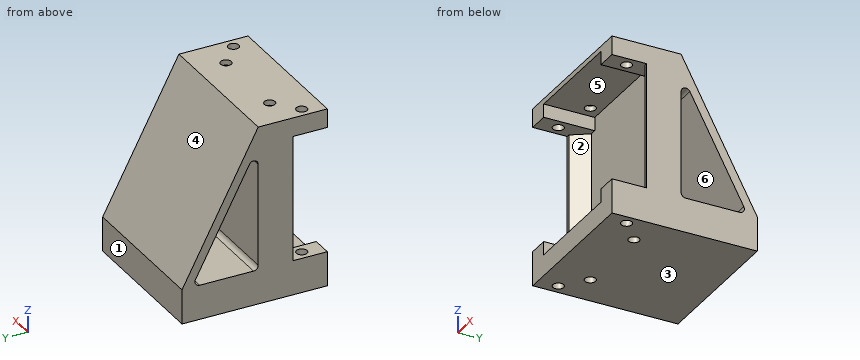
from build123d import *

# Parameters (mm, degrees)
BOSS_EXTRUDE1_DEPTH = 40.132
FILLET1_R           = 1.27
SKETCH2_W           = 28.2956
SKETCH2_H           = 34.036
CUT_EXTRUDE1_DEPTH  = 4.4704
CHAMFER1_SIZE       = 5.08
CHAMFER1_SIZE_2     = 7.53140972
SKETCH3_R           = 1.4605
CUT_EXTRUDE2_DEPTH  = 73.627884767
CUT_EXTRUDE4_REACH  = 76.199
SKETCH4_W           = 28.956
SKETCH4_H           = 41.3004


with BuildPart() as part:
    # Sketch1 → Boss-Extrude1 (new body)
    with BuildSketch(Plane(origin=(0, 0, 0), x_dir=(0, 0, -1), z_dir=(1, 0, 0))):
        Polygon((0, -3.052283086), (0, 36.270517883), (-9.3472, 36.270517883), (-48.4632, 15.642116914), (-48.4632, -3.052283086), (-43.3832, -3.052283086), (-43.3832, 6.294916914), (-9.3472, 6.294916914), (-9.3472, -3.052283086), align=None)
        Polygon((-43.3832, 15.642116914), (-9.3472, 33.59150477), (-9.3472, 15.642116914), align=None, mode=Mode.SUBTRACT)
    extrude(amount=BOSS_EXTRUDE1_DEPTH)

    # Fillet1
    fillet1_edges = [part.edges().sort_by_distance(p)[0] for p in [
        (20.066, 15.642116914, 43.3832),
        (20.066, 15.642116914, 9.3472),
        (20.066, 33.59150477, 9.3472),
    ]]
    fillet(fillet1_edges, radius=FILLET1_R)

    # Sketch2 → Cut-Extrude1 (cut)
    with BuildSketch(Plane.XZ.offset(-6.294916914)):
        with Locations((20.066, 26.3652)):
            Rectangle(SKETCH2_W, SKETCH2_H)
    extrude(amount=-CUT_EXTRUDE1_DEPTH, mode=Mode.SUBTRACT)

    # Chamfer1
    # the kernel refuses this chamfer: 7.53140972, 5.08 mm, written as the material it takes off along each edge
    with BuildSketch(Plane(origin=(5.9182, 6.294916914, 9.3472), x_dir=(-0.9988697089125115, -0.04753214298802862, 0), z_dir=(0, 0, 1))) as chamfer1_piece_1_section:
        Polygon((CHAMFER1_SIZE * 0.998869708913, -CHAMFER1_SIZE * 0.047532142988), (-CHAMFER1_SIZE_2 * 0.0475321429883, -CHAMFER1_SIZE_2 * 0.998869708918), (0, 0), align=None)
    chamfer1_piece_1 = extrude(amount=34.036, mode=Mode.PRIVATE)
    chamfer1_piece_1 = split(chamfer1_piece_1, bisect_by=Plane(origin=(4.025982399, 10.765316914, 26.3652), z_dir=(0, -1, 0)), keep=Keep.TOP, mode=Mode.PRIVATE)
    add(chamfer1_piece_1, mode=Mode.SUBTRACT)
    with BuildSketch(Plane(origin=(34.2138, 6.294916914, 43.3832), x_dir=(0.9988697089125117, -0.0475321429880285, 0), z_dir=(0, 0, -1))) as chamfer1_piece_2_section:
        Polygon((CHAMFER1_SIZE * 0.998869708913, -CHAMFER1_SIZE * 0.047532142988), (-CHAMFER1_SIZE_2 * 0.0475321429883, -CHAMFER1_SIZE_2 * 0.998869708918), (0, 0), align=None)
    chamfer1_piece_2 = extrude(amount=34.036, mode=Mode.PRIVATE)
    chamfer1_piece_2 = split(chamfer1_piece_2, bisect_by=Plane(origin=(36.106017601, 10.765316914, 26.3652), z_dir=(0, -1, 0)), keep=Keep.TOP, mode=Mode.PRIVATE)
    add(chamfer1_piece_2, mode=Mode.SUBTRACT)

    # Sketch3 → Cut-Extrude2 (cut, through all)
    with BuildSketch(Plane(origin=(0, 0, 0), x_dir=(-1, 0, 0), z_dir=(0, 0, -1))):
        with Locations((-37.338, 2.383316914)):
            Circle(SKETCH3_R)
        with Locations((-31.115, 7.717316914)):
            Circle(SKETCH3_R)
        with Locations((-9.017, 7.717316914)):
            Circle(SKETCH3_R)
        with Locations((-2.794, 2.383316914)):
            Circle(SKETCH3_R)
    extrude(amount=-CUT_EXTRUDE2_DEPTH, mode=Mode.SUBTRACT)

    # Cut-Extrude4: up to this face of the body (flat: up to its plane)
    cut_extrude4_end = Plane(part.part.faces().sort_by_distance((20.066, 10.765316914, 26.3652))[0])
    # Sketch4 → Cut-Extrude4 (cut, up to the picked face)
    with BuildSketch(Plane.XZ.offset(3.052283086), mode=Mode.PRIVATE) as cut_extrude4_sk1:
        with Locations((20.066, 26.3652)):
            Rectangle(SKETCH4_W, SKETCH4_H)
    cut_extrude4_tool1 = split(extrude(cut_extrude4_sk1.sketch, amount=-CUT_EXTRUDE4_REACH, mode=Mode.PRIVATE), bisect_by=cut_extrude4_end, keep=Keep.BOTH, mode=Mode.PRIVATE)
    add(cut_extrude4_tool1.solids().sort_by(Axis((20.066, -3.052283, 26.3652), (0, 1, 0)))[0], mode=Mode.SUBTRACT)


solid = part.part
The listing builds one solid part. Answer for the finished solid, in the listing's coordinates (mm). Face numbers are marked on the shaded views. A direction names the side the tool comes from. Give positions to 0.01 mm unless a question says otherwise; leave off trailing zeros. Loops run counter-clockwise (first coordinate to the right, second up) from the corner with the lowest first, then second, coordinate; pieces in that order, holes last. Notation, with made-up numbers: (25.5, 76.25) - (80.5, 76.25) arc R13 cw to (80.5, 99.25) - close; hole circle Ø9 at (19, 80). An arc over 180 degrees is marked (long way). Write each question's results on one line, items separated by ' | '.
1. For a pull along Z with two mould halves and no side action, classify the marked faces 1, 2 and 3 as +Z half, -Z half, draft (parallel to the pull), parting line (faces both ways), or undercut.
Resolved:
face 1: draft | face 2: undercut | face 3: -Z half
2. Consider probe 1 along Z at (x, y) = (27.5, 9) (3 decimals); probe 2 along Y at (x, z) = (15.5, 22); probe 3 along Y at (x, z) = (13, 6). Determine where each line is inside the solid, lowest interval first. Write a range as from..to.
Resolved:
probe 1: z = 0..5.715, 47.015..48.463 | probe 2: y = 10.77..15.64, 26.92..29.6 | probe 3: y = 10.77..36.27
3. Flat-ended cylindrical pins translate along their axes: P1, Ø0.9, axis at x = 39.5, z = 31, coming from the -Y side; P2, Ø8.5, axis at x = 26.5, z = 31, coming from the +Y side; P3, Ø16, axis at x = 22, y = 25, coming from the +Z side. Find the tip coordinate at first contact, or state that the pin passes through.
Resolved:
P1: stops at y = 6.29 | P2: stops at y = 27.09 | P3: stops at z = 45.89
4. Find section C-C, the plane y = 21.5. Write down the section's boundary in (x, z), then the cut area to 3 significant figures.
Resolved:
outline: (0, 0) - (40.13, 0) - (40.13, 9.35) - (0, 9.35) - close; (0, 32.28) - (40.13, 32.28) - (40.13, 37.36) - (0, 37.36) - close | area: 579 mm^2
5. Find section A-A, the plane x = 18.5. Write down the section's boundary in (y, z) (3 decimals), then the cut area to 3 significant figures.
Resolved:
outline: (-3.052, 0) - (36.271, 0) - (36.271, 9.347) - (15.642, 48.463) - (-3.052, 48.463) - (-3.052, 47.015) - (10.765, 47.015) - (10.765, 5.715) - (-3.052, 5.715) - close; hole (15.642, 10.617) arc R1.27 ccw to (16.912, 9.347) - (31.486, 9.347) arc R1.27 ccw to (32.609, 11.21) - (18.035, 38.845) arc R1.27 ccw to (15.642, 38.252) - close | area: 632 mm^2
6. Which of the six approach directions +Z, -Z, +X, -X, +Y, -Y give full straight-line access (tool end or side, diameter ignored) to the marked faces 4, 5 and 6?
Resolved:
face 4: +Z, +X, -X, +Y | face 5: -Y | face 6: +X, -X
7. Find section B-B, the plane z = 37.5. Write down the section's boundary in (x, y).
Resolved:
outline: (0, 6.29) - (0.84, 6.29) - (3.85, 10.77) - (36.28, 10.77) - (39.29, 6.29) - (40.13, 6.29) - (40.13, 15.64) - (0, 15.64) - close; (0, 18.74) - (40.13, 18.74) - (40.13, 21.42) - (0, 21.42) - close
